Autodesk Inventor part; units mm, degrees
ref_plane "YZ Plane" through (0, 0, 0) normal (1, 0, 0) x (0, 1, 0)
ref_plane "XZ Plane" through (0, 0, 0) normal (0, 1, 0) x (-1, 0, 0)
ref_plane "XY Plane" through (0, 0, 0) normal (0, 0, 1) x (1, 0, 0)
sketch "Sketch1" plane through (0, 0, 0) normal (0, 1, 0) x (-1, 0, 0)
  circle A0 centre (0, 0) radius 9
  dimension "d0" = 18
extrude "Extrusion1" add sketch "Sketch1" along normal blind 23.5
sketch "Sketch2" plane through (0, 23.5, 0) normal (0, 1, 0) x (1, 0, 0)
  circle A0 centre (0, 0) radius 5.5
  dimension "d3" = 11
extrude "Extrusion2" cut sketch "Sketch2" against normal up to next
sketch "Sketch3" plane through (0, 23.5, 0) normal (0, 1, 0) x (1, 0, 0)
  circle A0 centre (0, 0) radius 1.75
  circle A1 centre (0, 0) radius 9
  dimension "d6" = 3.5
  dimension "d7" = 18
extrude "Extrusion3" add sketch "Sketch3" against normal blind 15.5
properties part number "Idle_Pulley_Bearing"
Work out the finished part from the listing and answer in its coordinate system (mm). A direction names the side the tool comes from. Coordinates: 2 decimals unless noted, no trailing zeros. Loops run counter-clockwise (first coordinate to the right, second up) from the corner with the lowest first, then second, coordinate; pieces in that order, holes last. Notation, with made-up numbers: M 68,-15 L 118,-15 A11 ccw 118,2 Z; hole C 50.25,11 d5. An arc over 180 degrees is marked long. Answer in a Markdown table with one row per item. Add a question column.
1. Find section D-D, the plane x = -3.5. Write down the section's boundary in (y, z), then the cut area to 3 significant figures.
2. The mould has two halves that part along Z. Classify faces 3 (the cylindrical face through (1.172, 11.586, -8.923)), 4 (the cylindrical face through (-1.19, 4.06, 5.37)), 5 (the flat face through (0, 23.5, -2)): pulls with the +Z half, pulls with the -Z half, needs draft (parallel to the pull), parting line crosses it, or undercut.
3. Find section A-A, the plane z = 0. Write down the section's boundary in (x, y).
4. A tool of negligible diameter and unlimited length cuts with its end or side. For faces 1 (the flat face through (4, 0, -4)), 2 (the flat face through (0, 8, 2)), from which of +Z, -Z, +X, -X, +Y, -Y can it reach the whole face along a straight path? Write none if from no direction.
5. Find section C-C, the plane y = 4.25. Write down the section's boundary in (x, z).
6. Flat-ended cylindrical pins translate along their axes: P1, Ø1, axis at x = -6.5, y = 16, coming from the +Z side; P2, Ø3, axis at x = -5, y = 20.5, coming from the -Z side; P3, Ø3.5, axis at x = -0.5, z = -0.5, coming from the -Y side. Find the tip coordinate at first contact, or state that the pin passes through.
7. Consider L1, parallel to X at y = 12.25, z = 0; L2, parallel to Z at x = 0, y = 4.25. Determine where each line is inside the solid, lowest interval first.
8. Find section B-B, the plane x = 0. Write down the section's boundary in (y, z).
Reported:
| question | item | result |
|---|---|---|
| 1 | outline | M 0,-8.29 L 23.5,-8.29 L 23.5,8.29 L 0,8.29 L 0,4.24 L 8,4.24 L 8,-4.24 L 0,-4.24 Z |
| 1 | area | 322 mm^2 |
| 2 | face 3 | parting line crosses it |
| 2 | face 4 | undercut |
| 2 | face 5 | needs draft |
| 3 | outline | M -9,0 L -5.5,0 L -5.5,8 L -1.75,8 L -1.75,23.5 L -9,23.5 Z; M 1.75,8 L 5.5,8 L 5.5,0 L 9,0 L 9,23.5 L 1.75,23.5 Z |
| 4 | face 1 | +Z, -Z, +X, -X, -Y |
| 4 | face 2 | -Y |
| 5 | outline | C 0,0 d18; hole C 0,0 d11 |
| 6 | P1 | stops at z = 6.71 |
| 6 | P2 | stops at z = -8.29 |
| 6 | P3 | stops at y = 8 |
| 7 | L1 | x = -9 to -1.75, 1.75 to 9 |
| 7 | L2 | z = -9 to -5.5, 5.5 to 9 |
| 8 | outline | M 0,-9 L 23.5,-9 L 23.5,-1.75 L 8,-1.75 L 8,-5.5 L 0,-5.5 Z; M 0,5.5 L 8,5.5 L 8,1.75 L 23.5,1.75 L 23.5,9 L 0,9 Z |
